Source: CAD feature listing. Evaluate the final solid. Frame: model axes, mm. Face numbers are marked on the shaded views. Give positions to 0.01 mm unless a question says otherwise; leave off trailing zeros. Write each loop counter-clockwise with the first axis right and the second up, starting at its lowest first coordinate (ties: lowest second). Pieces come first, ordered by that corner, then holes. Notation, with made-up numbers: (-3, 56) -> (43, 56) arc R31 cw to (43, 82) -> close; hole circle Ø2 at (-21, 22.25). An arc over 180 degrees is marked (long way). Write item = value, one per line.
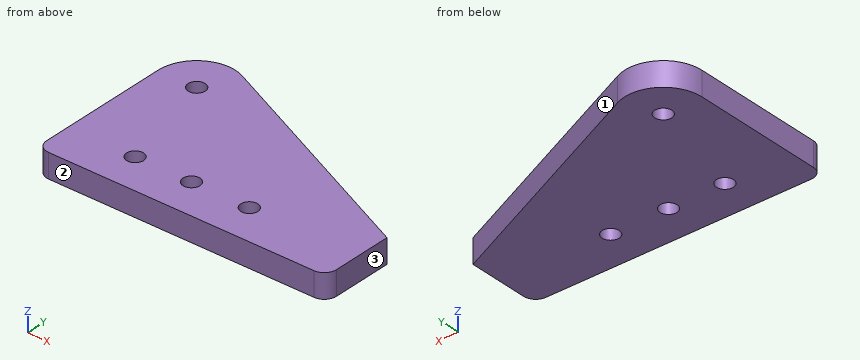
Autodesk Inventor part; units mm, degrees
ref_plane "YZ Plane" through (0, 0, 0) normal (1, 0, 0) x (0, 1, 0)
ref_plane "XZ Plane" through (0, 0, 0) normal (0, 1, 0) x (-1, 0, 0)
ref_plane "XY Plane" through (0, 0, 0) normal (0, 0, 1) x (1, 0, 0)
sketch "Sketch1" plane through (0, 0, 0) normal (0, 0, 1) x (1, 0, 0)
  line L0 (38.1, -19.05) -> (-38.1, -19.05)
  line L1 (-38.1, -19.05) -> (-38.1, 19.05)
  line L2 (-38.1, 19.05) -> (38.1, 19.05)
  line L3 (38.1, 19.05) -> (38.1, -19.05)
  line L4 (38.1, -19.05) -> (-38.1, 19.05) construction
  line L5 (-38.1, -19.05) -> (38.1, 19.05) construction
  line L6 (-38.1, -19.05) -> (38.1, -19.05)
  line L7 (38.1, -19.05) -> (38.1, 0.8382)
  line L8 (38.1, 0.8382) -> (-38.1, 0.8382) construction
  line L9 (-38.1, 0.8382) -> (-38.1, -19.05)
  line L10 (-38.1, -9.1059) -> (38.1, -9.1059) construction
  circle A0 centre (-20.5232, -9.1059) radius 2.25
  circle A1 centre (-5.6896, -9.1059) radius 2.25
  circle A2 centre (9.525, -9.1059) radius 2.25
  circle A3 centre (-27.94, 19.05) radius 6.35 construction
  circle A4 centre (-27.94, 19.05) radius 2.25
  circle A5 centre (-27.94, 19.05) radius 10.16
  line L11 (38.1, 0) -> (-23.712, 28.2885)
  point P0 (0, 0)
  point P1 (-38.1, 19.05)
  point P2 (-17.78, 19.05)
  point P3 (-3.5254, 19.05)
  dimension "d0" = 76.2
  dimension "d1" = 38.1
  dimension "d2" = 19.8882
  dimension "d3" = 4.5
  dimension "d4" = 17.5768
  dimension "d5" = 4.5
  dimension "d6" = 14.8336
  dimension "d7" = 4.5
  dimension "d8" = 15.2146
  dimension "d9" = 12.7
  dimension "d10" = 0
  dimension "d11" = 10.16
  dimension "d12" = 4.5
extrude "Extrusion1" add sketch "Sketch1" along normal blind 6.35 contours L0 L1 A5 L2 L11 L3 | L11 L2 L3 | L2 A5 L11 | A5 L2 A4 | L2 A4 A5
extrude "Extrusion2" cut sketch "Sketch1" along normal blind 6.35 contours L11 L2 L3
fillet "Fillet1" radius 3.175 2 edges at (38.1, -19.05, 3.175) (-38.1, -19.05, 3.175)
properties part number "Slide_Climb_Conforce_Spring_Mount"
1) Cut plane C-C (z = 4). State how many separate pieces and enclosed holes the cut face has, then the cut area to 3 significant figures.
Computed:
separate_pieces = 1
enclosed_holes = 4
area = 2,650 mm²
2) Draft query along Y for the marked faces 1, 2 and 3. Return one class per face: pulls with the +Y half, pulls with the -Y half, needs draft (parallel to the pull), parting line crosses it, or undercut.
Computed:
face_1 = pulls with the +Y half
face_2 = pulls with the -Y half
face_3 = needs draft
3) Cut plane A-A (x = -27.94). Return the cut outline in (y, z), then the cut area to 3 significant figures.
Computed:
outline = (-19.05, 0) -> (16.8, 0) -> (16.8, 6.35) -> (-19.05, 6.35) -> close; (21.3, 0) -> (29.21, 0) -> (29.21, 6.35) -> (21.3, 6.35) -> close
area = 278 mm²
4) Cut plane D-D (x = 32). Return the cut outline in (y, z), then the cut area to 3 significant figures.
Computed:
outline = (-19.05, 0) -> (2.79, 0) -> (2.79, 6.35) -> (-19.05, 6.35) -> close
area = 139 mm²
5) Cut plane B-B (y = -10). Return the cut outline in (x, z), then the cut area to 3 significant figures.
Computed:
outline = (-38.1, 0) -> (-22.59, 0) -> (-22.59, 6.35) -> (-38.1, 6.35) -> close; (-18.46, 0) -> (-7.75, 0) -> (-7.75, 6.35) -> (-18.46, 6.35) -> close; (-3.62, 0) -> (7.46, 0) -> (7.46, 6.35) -> (-3.62, 6.35) -> close; (11.59, 0) -> (38.1, 0) -> (38.1, 6.35) -> (11.59, 6.35) -> close
area = 405 mm²
6) Contact query for flat-ended pins moving along their axis: pin 1 (4 mm diameter, centred on x = 9.52, y = -9.11, fed in from +Z); pin 2 (3 mm diameter, centred on y = 9.5, z = 3.5, fed in from +X). Output: stop coordinate, or through.
Computed:
pin_1 = through
pin_2 = 20.62
7) Material intervals for L1, parallel to X at y = -10, z = 1.5; L2, parallel to X at y = 19.05, z = 2.25; L3, parallel to X at y = -8, z = 1, sorted ascending.
Computed:
L1 = -38.1 to -22.59, -18.46 to -7.75, -3.62 to 7.46, 11.59 to 38.1
L2 = -38.1 to -30.19, -25.69 to -3.53
L3 = -38.1 to -22.48, -18.56 to -7.65, -3.73 to 7.57, 11.48 to 38.1
